Work out the finished part from the listing and answer in its coordinate system (mm). Face numbers are marked on the shaded views. A direction names the side the tool comes from. Coordinates: 2 decimals unless noted, no trailing zeros. Loops run counter-clockwise (first coordinate to the right, second up) from the corner with the lowest first, then second, coordinate; pieces in that order, holes last. Notation, with made-up numbers: (16.5, 24.5) -> (63.5, 24.5) arc R30 ccw to (63.5, 50.5) -> close; hole circle Ø7 at (83, 51). An arc over 180 degrees is marked (long way). Answer as CSV lines item,"result".
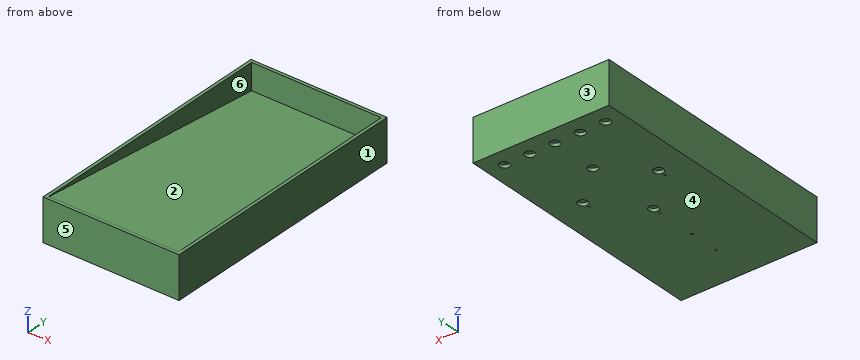
```python
from build123d import *

# Parameters (mm, degrees)
F0_R     = 6.35
F0_R_2   = 29
F1_DEPTH = 19.05
F0_W     = 820
F0_H     = 1562.1
F2_DEPTH = 254
F4_DEPTH = 819.9882


with BuildPart() as f1:
    # F0 (on Top) → F1 (new body)
    with BuildSketch(Plane.XY):
        with BuildLine():
            Line((-357.9300045967, 709.0338208199), (-357.9300045967, -441.2995662034))
            Line((-357.9300045967, -441.2995662034), (-38.1, -557.7961837769))
            ThreePointArc((-38.1, -557.7961837769), (0, -519.6961837769), (38.1, -557.7961837769))
            Line((38.1, -557.7961837769), (357.9300045967, -441.2995662034))
            Line((357.9300045967, -441.2995662034), (357.9300045967, 709.0338208199))
            Line((357.9300045967, 709.0338208199), (-357.9300045967, 709.0338208199))
        make_face()
        with Locations((0, -373.6461837769)):
            Circle(F0_R, mode=Mode.SUBTRACT)
        with Locations((0, -132.3461837769)):
            Circle(F0_R, mode=Mode.SUBTRACT)
        with Locations((0, -84.2961837769)):
            Circle(F0_R_2, mode=Mode.SUBTRACT)
        with Locations((-228.5999953747, 114.8538155079)):
            Circle(F0_R, mode=Mode.SUBTRACT)
        with Locations((-228.6, 162.9038156998)):
            Circle(F0_R_2, mode=Mode.SUBTRACT)
        with Locations((-304.8, 655.9038162231)):
            Circle(F0_R_2, mode=Mode.SUBTRACT)
        with Locations((-152.4, 655.9038162231)):
            Circle(F0_R_2, mode=Mode.SUBTRACT)
        with Locations((228.5999959257, 114.8538155079)):
            Circle(F0_R, mode=Mode.SUBTRACT)
        with Locations((228.6, 162.9038155079)):
            Circle(F0_R_2, mode=Mode.SUBTRACT)
        with Locations((0, 372.9038162231)):
            Circle(F0_R_2, mode=Mode.SUBTRACT)
        with Locations((0, 655.9038162231)):
            Circle(F0_R_2, mode=Mode.SUBTRACT)
        with Locations((152.4, 655.9038162231)):
            Circle(F0_R_2, mode=Mode.SUBTRACT)
        with Locations((304.8, 655.9038162231)):
            Circle(F0_R_2, mode=Mode.SUBTRACT)
        Polygon((357.9300045967, -557.7961837769), (357.9300045967, -441.2995662034), (38.1, -557.7961837769), align=None)
        Polygon((-38.1, -557.7961837769), (-357.9300045967, -441.2995662034), (-357.9300045967, -557.7961837769), align=None)
        with BuildLine():
            Line((-38.1, -557.7961837769), (-357.9300045967, -557.7961837769))
            Line((-357.9300045967, -557.7961837769), (-357.9300045967, -748.9261883736))
            Line((-357.9300045967, -748.9261883736), (357.9300045967, -748.9261883736))
            Line((357.9300045967, -748.9261883736), (357.9300045967, -557.7961837769))
            Line((357.9300045967, -557.7961837769), (38.1, -557.7961837769))
            Line((38.1, -557.7961837769), (6.35, -557.7961837769))
            ThreePointArc((6.35, -557.7961837769), (0, -564.1461837769), (-6.35, -557.7961837769))
            Line((-6.35, -557.7961837769), (-38.1, -557.7961837769))
        make_face()
        with BuildLine():
            ThreePointArc((38.1, -557.7961837769), (0, -519.6961837769), (-38.1, -557.7961837769))
            Line((-38.1, -557.7961837769), (-6.35, -557.7961837769))
            ThreePointArc((-6.35, -557.7961837769), (0, -551.4461837769), (6.35, -557.7961837769))
            Line((6.35, -557.7961837769), (38.1, -557.7961837769))
        make_face()
        Polygon((390.95, 742.0538162231), (-390.95, 742.0538162231), (-390.95, -429.2721837769), (-357.9300045967, -441.2995662034), (-357.9300045967, 709.0338208199), (357.9300045967, 709.0338208199), (357.9300045967, -441.2995662034), (390.95, -429.2721837769), align=None)
        Polygon((-357.9300045967, -441.2995662034), (-390.95, -429.2721837769), (-390.95, -557.7961837769), (-357.9300045967, -557.7961837769), align=None)
        Polygon((-357.9300045967, -557.7961837769), (-390.95, -557.7961837769), (-390.95, -781.9461837769), (390.95, -781.9461837769), (390.95, -557.7961837769), (357.9300045967, -557.7961837769), (357.9300045967, -748.9261883736), (-357.9300045967, -748.9261883736), align=None)
        Polygon((390.95, -557.7961837769), (390.95, -429.2721837769), (357.9300045967, -441.2995662034), (357.9300045967, -557.7961837769), align=None)
    extrude(amount=F1_DEPTH)

    # F0 (on Top) → F2 (join)
    with BuildSketch(Plane.XY):
        with Locations((0, -19.9461837769)):
            Rectangle(F0_W, F0_H)
        Polygon((-390.95, -429.2721837769), (-390.95, 742.0538162231), (390.95, 742.0538162231), (390.95, -429.2721837769), (390.95, -557.7961837769), (390.95, -781.9461837769), (-390.95, -781.9461837769), (-390.95, -557.7961837769), align=None, mode=Mode.SUBTRACT)
    extrude(amount=F2_DEPTH)

    # F3 (on face) → F4 (join)
    with BuildSketch(Plane.YZ.offset(410)):
        Polygon((-800.9961837769, 234.95), (761.1038162231, 76.2), (761.1038162231, 95.25), (-800.9961837769, 254), align=None)
    extrude(amount=-F4_DEPTH)


solid = f1.part
```
(1) Consider line 1 along Y through (x, z) = (228, 14); line 2 along X through (y, z) = (-516, 48); line 3 along Y through (x, z) = (-362.5, 46). Determine where each line is inside the solid, lowest interval first.
Computed values:
line 1,"-801 to 108.53, 121.18 to 133.91, 191.9 to 761.1"
line 2,"-410 to -390.95, 390.95 to 410"
line 3,"-801 to -781.95, 742.05 to 761.1"
(2) A cutting plane is placed at D-D, the plane x = 301.5. Write down the section's boundary in (y, z), and give its area (3 significant figures).
Computed values:
outline,"(-801, 0) -> (627.09, 0) -> (627.09, 19.05) -> (-781.95, 19.05) -> (-781.95, 233.01) -> (742.05, 78.14) -> (742.05, 19.05) -> (684.72, 19.05) -> (684.72, 0) -> (761.1, 0) -> (761.1, 254) -> (742.05, 254) -> (742.05, 97.19) -> (-781.95, 252.06) -> (-781.95, 254) -> (-801, 254) -> close"
area,"66,600 mm2"
(3) Flat-ended cylindrical pins translate along their axes: pin 1 Ø4 at (x, y) = (77.5, 55) entering from -Z; pin 2 Ø7.5 at (x, y) = (0, -373.65) entering from +Z; pin 3 Ø7.5 at (x, y) = (0, -132.35) entering from +Z. Find the tip coordinate at first contact, or state that the pin passes through.
Computed values:
pin 1,"z = 0"
pin 2,"z = 210.95"
pin 3,"z = 186.43"
(4) A cutting plane is placed at B-B, the plane x = -152.4. Write down the section's boundary in (y, z), and give its area (3 significant figures).
Computed values:
outline,"(-801, 0) -> (626.9, 0) -> (626.9, 19.05) -> (-781.95, 19.05) -> (-781.95, 233.01) -> (742.05, 78.14) -> (742.05, 19.05) -> (684.9, 19.05) -> (684.9, 0) -> (761.1, 0) -> (761.1, 254) -> (742.05, 254) -> (742.05, 97.19) -> (-781.95, 252.06) -> (-781.95, 254) -> (-801, 254) -> close"
area,"66,600 mm2"
(5) A cutting plane is placed at C-C, the plane y = -289. Write down the section's boundary in (x, z).
Computed values:
outline,"(-410, 0) -> (410, 0) -> (410, 254) -> (390.95, 254) -> (390.95, 201.97) -> (-390.95, 201.97) -> (-390.95, 254) -> (-410, 254) -> close; hole (-390.95, 19.05) -> (390.95, 19.05) -> (390.95, 182.92) -> (-390.95, 182.92) -> close"
(6) A cutting plane is placed at A-A, the plane z = 46.5. Write down the section's boundary in (x, y), and give its area (3 significant figures).
Computed values:
outline,"(-410, -801) -> (410, -801) -> (410, 761.1) -> (-410, 761.1) -> close; hole (-390.95, -781.95) -> (390.95, -781.95) -> (390.95, 742.05) -> (-390.95, 742.05) -> close"
area,"89,300 mm2"
(7) For a pull along Y with two mould halves and no side action, classify the marked faces 3, 4, 5 and 6 as pulls with the +Y half, pulls with the -Y half, needs draft (parallel to the pull), parting line crosses it, or undercut.
Computed values:
face 3,"pulls with the +Y half"
face 4,"needs draft"
face 5,"pulls with the -Y half"
face 6,"undercut"
(8) Which of the six approach directions +Z, -Z, +X, -X, +Y, -Y give full straight-line access (tool end or side, diameter ignored) to the marked faces 1 and 2?
Computed values:
face 1,"+Z, -Z, +X, +Y, -Y"
face 2,"+Z"
